The listing builds one solid part. Answer for the finished solid, in the listing's coordinates (mm). Face numbers are marked on the shaded views. A direction names the side the tool comes from. Coordinates: 2 decimals unless noted, no trailing zeros. Order: outer loops, then holes, each group sorted by start corner. A loop starts at its lowest first (then second) coordinate and runs counter-clockwise, first axis right, second up. Notation, with made-up numbers: (28, 57.5) -> (42, 57.5) arc R22 ccw to (42, 84.5) -> close; hole circle Ø6 at (30, 64). An arc over 180 degrees is marked (long way). Answer in a Markdown table with one row per item. Add a question column.
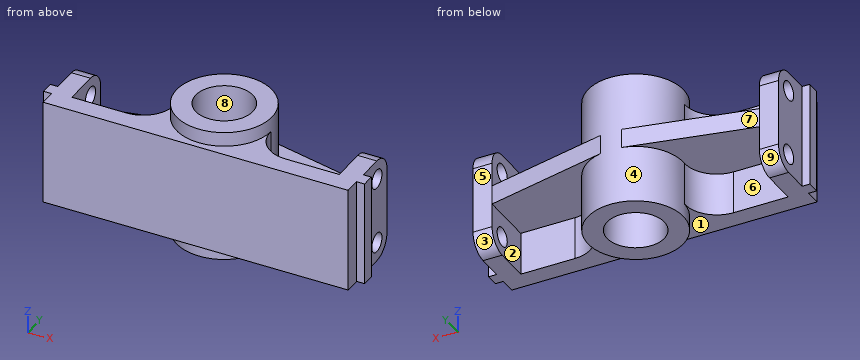
```python
from build123d import *

# Parameters (mm, degrees)
SKETCH1_R                      = 30
SKETCH1_R_2                    = 18
BOSS_EXTRUDE1_DEPTH            = 84
BOSS_EXTRUDE3_DEPTH            = 66
CUT_EXTRUDE1_REACH             = 218.843
SKETCH3_R                      = 6
CUT_EXTRUDE1_DIRECTION_2_DEPTH = 217.843261366
FILLET1_R                      = 12
CUT_EXTRUDE2_REACH             = 219.029
SKETCH4_R                      = 6
FILLET2_R                      = 12
RIB1_REACH                     = 116.547
SKETCH5_WALL_W                 = 310.682445014
SKETCH5_WALL_H                 = 12
RIB2_REACH                     = 116.547
SKETCH6_WALL_W                 = 310.466406556
SKETCH6_WALL_H                 = 12


with BuildPart() as part:
    # Sketch1 → Boss-Extrude1 (new body)
    with BuildSketch(Plane.XY):
        with Locations(Location((0, 0, 0), (0, 0, 180))):
            Circle(SKETCH1_R)
        with Locations(Location((0, 0, 0), (0, 0, 180))):
            Circle(SKETCH1_R_2, mode=Mode.SUBTRACT)
    extrude(amount=BOSS_EXTRUDE1_DEPTH)

    # Sketch2 → Boss-Extrude3 (add)
    with BuildSketch(Plane.XY.offset(9)):
        with BuildLine():
            Line((96, -24), (101, -24))
            Line((101, -24), (101, -16))
            Line((101, -16), (96, -16))
            Line((96, -16), (96, 12))
            Line((96, 12), (84, 12))
            Line((84, 12), (84, -22))
            Line((84, -22), (49.959983987, -22))
            ThreePointArc((49.959983987, -22), (35.537778885, -15.856406461), (29.975990392, -1.2))
            ThreePointArc((29.975990392, -1.2), (0, -30), (-29.975990392, -1.2))
            ThreePointArc((-29.975990392, -1.2), (-35.537778885, -15.856406461), (-49.959983987, -22))
            Line((-49.959983987, -22), (-84.204166847, -22))
            Line((-84.204166847, -22), (-84.204166847, 12))
            Line((-84.204166847, 12), (-96.204166847, 12))
            Line((-96.204166847, 12), (-96.204166847, -16))
            Line((-96.204166847, -16), (-101, -16))
            Line((-101, -16), (-101, -24))
            Line((-101, -24), (-96, -24))
            Line((-96, -24), (-96, -34))
            Line((-96, -34), (96, -34))
            Line((96, -34), (96, -24))
        make_face()
    extrude(amount=BOSS_EXTRUDE3_DEPTH)

    # Sketch3 → Cut-Extrude1 (cut, up to next)
    with BuildSketch(Plane(origin=(96, 0, 0), x_dir=(0, 0, -1), z_dir=(1, 0, 0)), mode=Mode.PRIVATE) as cut_extrude1_sk1:
        with Locations(Location((-63, 0, 0), (0, 0, 180))):
            Circle(SKETCH3_R)
    cut_extrude1_tool1 = extrude(cut_extrude1_sk1.sketch, amount=-CUT_EXTRUDE1_REACH, mode=Mode.PRIVATE) & part.part
    # Sketch3 → Cut-Extrude1 (cut, up to next)
    with BuildSketch(Plane(origin=(96, 0, 0), x_dir=(0, 0, -1), z_dir=(1, 0, 0)), mode=Mode.PRIVATE) as cut_extrude1_sk2:
        with Locations(Location((-21, 0, 0), (0, 0, 180))):
            Circle(SKETCH3_R)
    cut_extrude1_tool2 = extrude(cut_extrude1_sk2.sketch, amount=-CUT_EXTRUDE1_REACH, mode=Mode.PRIVATE) & part.part
    add(cut_extrude1_tool1.solids().sort_by_distance((96, 0, 63))[0], mode=Mode.SUBTRACT)
    add(cut_extrude1_tool2.solids().sort_by_distance((96, 0, 21))[0], mode=Mode.SUBTRACT)

    # Sketch3 → Cut-Extrude1 direction 2 (cut)
    with BuildSketch(Plane(origin=(96, 0, 0), x_dir=(0, 0, -1), z_dir=(1, 0, 0))):
        with Locations(Location((-63, 0, 0), (0, 0, 180))):
            Circle(SKETCH3_R)
        with Locations(Location((-21, 0, 0), (0, 0, 180))):
            Circle(SKETCH3_R)
    extrude(amount=CUT_EXTRUDE1_DIRECTION_2_DEPTH, mode=Mode.SUBTRACT)

    # Fillet1
    fillet1_edges = [part.edges().sort_by_distance(p)[0] for p in [
        (90, 12, 9),
        (90, 12, 75),
    ]]
    fillet(fillet1_edges, radius=FILLET1_R)

    # Sketch4 → Cut-Extrude2 (cut, up to next)
    with BuildSketch(Plane.ZY.offset(96.204166847), mode=Mode.PRIVATE) as cut_extrude2_sk1:
        with Locations((21, 0)):
            Circle(SKETCH4_R)
    cut_extrude2_tool1 = extrude(cut_extrude2_sk1.sketch, amount=-CUT_EXTRUDE2_REACH, mode=Mode.PRIVATE) & part.part
    # Sketch4 → Cut-Extrude2 (cut, up to next)
    with BuildSketch(Plane.ZY.offset(96.204166847), mode=Mode.PRIVATE) as cut_extrude2_sk2:
        with Locations((63, 0)):
            Circle(SKETCH4_R)
    cut_extrude2_tool2 = extrude(cut_extrude2_sk2.sketch, amount=-CUT_EXTRUDE2_REACH, mode=Mode.PRIVATE) & part.part
    add(cut_extrude2_tool1.solids().sort_by_distance((-96.204167, 0, 21))[0], mode=Mode.SUBTRACT)
    add(cut_extrude2_tool2.solids().sort_by_distance((-96.204167, 0, 63))[0], mode=Mode.SUBTRACT)

    # Fillet2
    fillet2_edges = [part.edges().sort_by_distance(p)[0] for p in [
        (-90.204166847, 12, 9),
        (-90.204166847, 12, 75),
    ]]
    fillet(fillet2_edges, radius=FILLET2_R)

    # Sketch5 wall → Rib1 (add, up to next)
    with BuildSketch(Plane(origin=(-45.359592124, 20.642016154, 42), x_dir=(0.976134410289, 0.217167246725, 0), z_dir=(-0.217167246725, 0.976134410289, 0)), mode=Mode.PRIVATE) as rib1_sk1:
        Rectangle(SKETCH5_WALL_W, SKETCH5_WALL_H)
    rib1_tool1 = extrude(rib1_sk1.sketch, amount=-RIB1_REACH, mode=Mode.PRIVATE) - part.part
    add(rib1_tool1.solids().sort_by_distance((-45.359592124, 20.642016154, 42))[0])

    # Sketch6 wall → Rib2 (add, up to next)
    with BuildSketch(Plane(origin=(45.265686516, 20.640194383, 42), x_dir=(-0.976012958873, 0.217712434444, 0), z_dir=(-0.217712434444, -0.976012958873, 0)), mode=Mode.PRIVATE) as rib2_sk1:
        Rectangle(SKETCH6_WALL_W, SKETCH6_WALL_H)
    rib2_tool1 = extrude(rib2_sk1.sketch, amount=RIB2_REACH, mode=Mode.PRIVATE) - part.part
    add(rib2_tool1.solids().sort_by_distance((45.265686516, 20.640194383, 42))[0])


solid = part.part
```
Q1. Determine the mould class of the marked faces 6, 7, 8 and 9 for opening direction X: +X half, -X half, draft (parallel to the pull), parting line (faces both ways), or undercut.
Q2. Straight lines are drawn through the part: line 1 (X direction, y = -8, z = 50); line 2 (X direction, y = 9.5, z = 20); line 3 (Z direction, x = 44, y = -22). For each, find the intervals that lie inside material, in ascending order.
Q3. Given pin 1 (2 mm diameter, centred on x = 0, z = 65, fed in from +Y); pin 2 (12 mm diameter, centred on y = 15, z = 48.5, fed in from +X); pin 3 (2.5 mm diameter, centred on x = 98, z = 30, fed in from -Y), each flat-ended and moving along its own axis, determine where each tip first touches the part or whether it passes through.
Q4. A cutting plane is placed at A-A (z = 24). State how many separate pieces and enclosed holes the cut face has, then the cut area to 3 significant figures.
Q5. For the marked faces 1, 2, 3, 4 and 5, determine the directions among +Z, -Z, +X, -X, +Y, -Y from which every point of the face is accessible in a straight line to the end or side of a thin tool.
Q6. A cutting plane is placed at B-B (x = 0). Determine the outline of the cut face in (y, z), then the cut area to 3 significant figures.
Returned:
| question | item | result |
|---|---|---|
| 1 | face 6 | undercut |
| 1 | face 7 | -X half |
| 1 | face 8 | undercut |
| 1 | face 9 | draft |
| 2 | line 1 | x = -96.2 to -84.2, -30.88 to -16.12, 16.12 to 30.88, 84 to 96 |
| 2 | line 2 | x = -96.2 to -84.2, -28.46 to -15.29, 15.29 to 28.46, 84 to 96 |
| 2 | line 3 | z = 9 to 75 |
| 3 | pin 1 | stops at y = 30 |
| 3 | pin 2 | stops at x = 96 |
| 3 | pin 3 | stops at y = -24 |
| 4 | separate pieces | 3 |
| 4 | enclosed holes | 1 |
| 4 | area | 4,840 mm² |
| 5 | face 1 | -Z, -Y |
| 5 | face 2 | -Z, +Y |
| 5 | face 3 | -Z, +X, +Y |
| 5 | face 4 | none |
| 5 | face 5 | +Z, -Z, +X, +Y |
| 6 | outline | (-34, 9) -> (-30, 9) -> (-30, 0) -> (-18, 0) -> (-18, 84) -> (-30, 84) -> (-30, 75) -> (-34, 75) -> close; (18, 0) -> (30, 0) -> (30, 84) -> (18, 84) -> close |
| 6 | area | 2,280 mm² |
